Read the model definition and answer for the solid it produces. Units are mm, in the model's axes. Coordinates: 2 decimals unless noted, no trailing zeros. Loops run counter-clockwise (first coordinate to the right, second up) from the corner with the lowest first, then second, coordinate; pieces in that order, holes last. Notation, with made-up numbers: (76.25, 0.25) -> (111.25, 0.25) arc R35 ccw to (111.25, 33.25) -> close; hole circle Ø4 at (79, 14). An arc over 180 degrees is marked (long way). Answer as a JSON object with one key per item and string values. Group by question number.
Q1. The part is cut by section D-D on z = 1.15. State how many separate pieces and enclosed holes the cut face has, and give its area (3 significant figures).
Q2. The part is cut by section A-A on x = 0. Write down the section's boundary in (y, z), and give its area (3 significant figures).
Q3. The part is cut by section B-B on y = -8.5. Write down the section's boundary in (x, z).
Q4. Straight lines are drawn through the part: line 1 along Y through (x, z) = (-4, 0.4); line 2 along Y through (x, z) = (-8.5, 1.35); line 3 along X through (y, z) = (-35.5, 0.85). For each, find the intervals that lie inside material, in ascending order. Write a range as [from, to].
Q5. The part is cut by section C-C on x = -10.5. Write down the section's boundary in (y, z).
Q6. Each of these flat-tipped pins is pushed along its axis until it touches: P1, Ø8, axis at x = 0.5, y = 3.5, coming from the +Z side; P2, Ø2.5, axis at x = 9.5, y = -38, coming from the +Z side. Where does it stop, or does it pass through?
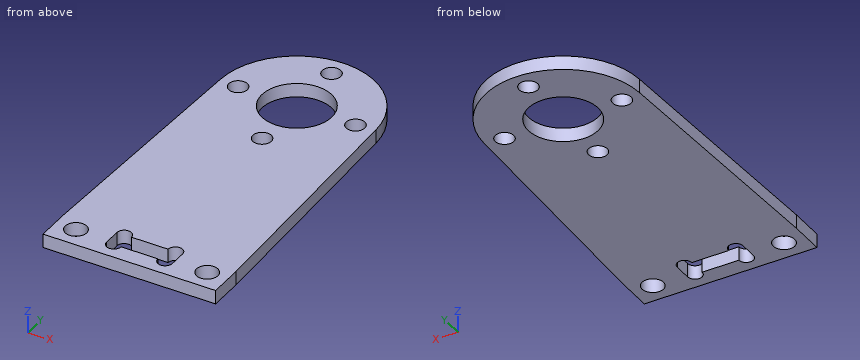
Autodesk Inventor part; units mm, degrees
ref_plane "YZ Plane" through (0, 0, 0) normal (1, 0, 0) x (0, 1, 0)
ref_plane "XZ Plane" through (0, 0, 0) normal (0, 1, 0) x (-1, 0, 0)
ref_plane "XY Plane" through (0, 0, 0) normal (0, 0, 1) x (1, 0, 0)
sketch "スケッチ1" plane through (0, 0, 0) normal (0, 0, 1) x (1, 0, 0)
  line L0 (-63.6765, 0) -> (66.53, 0) construction
  line L1 (0, 73.5962) -> (0, -63.7716) construction
  circle A0 centre (0, 0) radius 5.05
  circle A1 centre (0, 0) radius 8 construction
  circle A2 centre (0, 0) radius 11.25
  circle A3 centre (0, 8.5) radius 1.35
  circle A4 centre (0, 8.5) radius 2.75 construction
  circle A5 centre (-8.5, 0) radius 2.75 construction
  circle A6 centre (-8.5, 0) radius 1.35
  circle A7 centre (0, -8.5) radius 2.75 construction
  circle A8 centre (0, -8.5) radius 1.35
  circle A9 centre (8.5, 0) radius 2.75 construction
  circle A10 centre (8.5, 0) radius 1.35
  line L2 (12.5, -41) -> (-12.5, -41)
  line L3 (-12.5, -41) -> (-12.5, -36)
  line L4 (-12.5, -36) -> (12.5, -36) construction
  line L5 (12.5, -36) -> (12.5, -41)
  line L6 (12.5, -41) -> (-12.5, -36) construction
  line L7 (-12.5, -41) -> (12.5, -36) construction
  line L8 (12.5, -36) -> (11.2433, 0.3883)
  line L9 (-12.5, -36) -> (-11.2433, 0.3883)
  circle A11 centre (-9.5, -38) radius 1.55
  line L10 (-12.5, -38) -> (12.5, -38) construction
  line L11 (-4.75, -36) -> (-4.75, -41) construction
  line L12 (4.75, -36) -> (4.75, -41) construction
  circle A12 centre (9.5, -38) radius 1.55
  line L13 (-4.75, -36) -> (4.75, -36) construction
  line L14 (4.75, -36) -> (4.75, -38.5) construction
  line L15 (4.75, -38.5) -> (-4.75, -38.5) construction
  line L16 (-4.75, -38.5) -> (-4.75, -36) construction
  line L17 (-4.75, -37.25) -> (4.75, -37.25) construction
  line L18 (-4.76, -38.51) -> (4.76, -38.51)
  line L19 (4.76, -38.51) -> (4.76, -35.99)
  line L20 (4.76, -35.99) -> (-4.76, -35.99)
  line L21 (-4.76, -35.99) -> (-4.76, -38.51)
  circle A13 centre (-3.71, -35.99) radius 1.05
  circle A14 centre (-3.71, -38.51) radius 1.05
  circle A15 centre (3.71, -35.99) radius 1.05
  circle A16 centre (3.71, -38.51) radius 1.05
  point P0 (0, -38.5)
  point P1 (4.75, -36)
  point P2 (2.66, -38.51)
  point P3 (-2.66, -38.51)
  point P4 (-2.66, -35.99)
  point P5 (2.66, -35.99)
  dimension "d0" = 10.1
  dimension "d1" = 16
  dimension "d4" = 2.7
  dimension "d5" = 8.5
  dimension "d6" = 5.5
  dimension "d7" = 22.5
  dimension "d10" = 360
  dimension "d12" = 25
  dimension "d13" = 5
  dimension "d14" = 36
  dimension "d15" = 3
  dimension "d16" = 9.5
  dimension "d17" = 3.1
  dimension "d18" = 3
  dimension "d19" = 4.75
  dimension "d30" = 19
  dimension "d39" = 0.01
  dimension "d40" = 1.05
  dimension "d41" = 2.1
extrude "押し出し1" add sketch "スケッチ1" along normal blind 2
equation "\"d19\" = 0.5 * d16"
properties part number "Foot_roll_vertical_02" material "アルミニウム 2014-T4"
Final values:
{
 "1": {"separate pieces": "1", "enclosed holes": "8", "area": "1,030 mm2"},
 "2": {"outline": "(-41, 0) -> (-38.51, 0) -> (-38.51, 2) -> (-41, 2) -> close; (-35.99, 0) -> (-9.85, 0) -> (-9.85, 2) -> (-35.99, 2) -> close; (-7.15, 0) -> (-5.05, 0) -> (-5.05, 2) -> (-7.15, 2) -> close; (5.05, 0) -> (7.15, 0) -> (7.15, 2) -> (5.05, 2) -> close; (9.85, 0) -> (11.25, 0) -> (11.25, 2) -> (9.85, 2) -> close", "area": "68.5 mm2"},
 "3": {"outline": "(-11.55, 0) -> (-1.35, 0) -> (-1.35, 2) -> (-11.55, 2) -> close; (1.35, 0) -> (11.55, 0) -> (11.55, 2) -> (1.35, 2) -> close"},
 "4": {"line 1": "y = [-41, -39.52], [-34.98, -3.08], [3.08, 10.51]", "line 2": "y = [-41, -39.18], [-36.82, -1.35], [1.35, 7.37]", "line 3": "x = [-12.48, -4.64], [-2.78, 2.78], [4.64, 12.48]"},
 "5": {"outline": "(-41, 0) -> (-39.18, 0) -> (-39.18, 2) -> (-41, 2) -> close; (-36.82, 0) -> (4.04, 0) -> (4.04, 2) -> (-36.82, 2) -> close"},
 "6": {"P1": "stops at z = 2", "P2": "passes through"}
}
